Autodesk Inventor part; units mm, degrees
ref_plane "YZ Plane" through (0, 0, 0) normal (1, 0, 0) x (0, 1, 0)
ref_plane "XZ Plane" through (0, 0, 0) normal (0, 1, 0) x (-1, 0, 0)
ref_plane "XY Plane" through (0, 0, 0) normal (0, 0, 1) x (1, 0, 0)
sketch "Sketch1" plane through (0, 0, 0) normal (0, 1, 0) x (-1, 0, 0)
  line L0 (-25, -25) -> (25, -25)
  line L1 (25, -25) -> (25, 25)
  line L2 (25, 25) -> (-25, 25)
  line L3 (-25, 25) -> (-25, -25)
  line L4 (-25, -25) -> (25, 25) construction
  line L5 (25, -25) -> (-25, 25) construction
  point P0 (0, 0)
  dimension "d0" = 50
  dimension "d1" = 50
extrude "Extrusion1" add sketch "Sketch1" along normal blind 1
sketch "Sketch2" plane through (0, 1, 0) normal (0, 1, 0) x (1, 0, 0)
  line L0 (25, -25) -> (25, -15)
  line L1 (25, -25) -> (25, 25)
  line L2 (25, -15) -> (23.4, -15)
  line L3 (23.4, -15) -> (23.4, -5)
  line L4 (23.4, -5) -> (25, -5)
  line L5 (25, -5) -> (25, 5)
  line L6 (25, 5) -> (23.4, 5)
  line L7 (23.4, 5) -> (23.4, 15)
  line L8 (23.4, 15) -> (25, 15)
  line L9 (25, 15) -> (25, 25)
  line L10 (27, 25) -> (27, -25)
  line L11 (27, -25) -> (25, -25)
  point P0 (0, 0)
  dimension "d4" = 1.6
  dimension "d5" = 10
  dimension "d6" = 10
extrude "Extrusion2" cut sketch "Sketch2" against normal blind 1
sketch "Sketch3" plane through (0, 1, 0) normal (0, 1, 0) x (1, 0, 0)
  line L0 (25, 25) -> (25, 24)
  line L1 (25, 24) -> (15, 24)
  line L2 (15, 24) -> (15, 25)
  line L3 (25, 25) -> (-25, 25)
  line L4 (15, 25) -> (5, 25)
  line L5 (5, 25) -> (5, 24)
  line L6 (5, 24) -> (-5, 24)
  line L7 (-5, 24) -> (-5, 25)
  line L8 (-5, 25) -> (-15, 25)
  line L9 (-15, 25) -> (-15, 24)
  line L10 (-15, 24) -> (-25, 24)
  line L11 (-25, 24) -> (-25, 27)
  line L12 (-25, 27) -> (25, 27)
  line L13 (25, 27) -> (25, 25)
  point P0 (0, 0)
extrude "Extrusion3" cut sketch "Sketch3" against normal blind 1
sketch "Sketch4" plane through (0, 1, 0) normal (0, 1, 0) x (1, 0, 0)
  line L0 (-25, -25) -> (-25, -15)
  line L1 (-25, -15) -> (-24, -15)
  line L2 (-24, -15) -> (-24, -5)
  line L3 (-24, -5) -> (-25, -5)
  line L4 (-25, 24) -> (-25, -25)
  line L5 (-25, -5) -> (-25, 5)
  line L6 (-25, 24) -> (-25, -25)
  line L7 (-25, 5) -> (-24, 5)
  line L8 (-24, 5) -> (-24, 15)
  line L9 (-24, 15) -> (-25, 15)
  line L10 (-25, 24) -> (-27, 23)
  line L11 (-27, 23) -> (-27, -24.2648)
  line L12 (-27, -24.2648) -> (-25, -25)
  point P0 (0, 0)
  dimension "d11" = 10
  dimension "d12" = 10
  dimension "d13" = 10
extrude "Extrusion4" cut sketch "Sketch4" against normal blind 1 contours L4 L3 L2 L1 | L4 L9 L8 L7
sketch "Sketch5" plane through (0, 1, 0) normal (0, 1, 0) x (1, 0, 0)
  line L0 (-25, -25) -> (-15, -25)
  line L1 (-25, -25) -> (25, -25)
  line L2 (-15, -25) -> (-15, -24)
  line L3 (-15, -24) -> (-5, -24)
  line L4 (-5, -24) -> (-5, -25)
  line L5 (-5, -25) -> (5, -25)
  line L6 (5, -25) -> (5, -24)
  line L7 (5, -24) -> (15, -24)
  line L8 (15, -24) -> (15, -25)
  line L9 (25, -25) -> (25, -26)
  line L10 (25, -26) -> (-25, -26)
  line L11 (-25, -26) -> (-25, -25)
  point P0 (0, 0)
  dimension "d16" = 10
extrude "Extrusion5" cut sketch "Sketch5" against normal blind 1 contours L2 L3 L4 L1 | L6 L7 L8 L1
sketch "Sketch6" plane through (0, 1, 0) normal (0, 1, 0) x (1, 0, 0)
  circle A0 centre (-21.5, -18.2) radius 0.5
  circle A1 centre (-18.2, 21.5) radius 0.5
  circle A2 centre (18.2, -21.5) radius 0.5
  circle A3 centre (21.5, 18.2) radius 0.5
  line L0 (15, -25) -> (25, -25)
  line L1 (25, -25) -> (25, -15)
  line L2 (-25, -25) -> (-15, -25)
  line L3 (-25, -15) -> (-25, -25)
  line L4 (-5, 25) -> (-15, 25)
  line L5 (-25, 24) -> (-25, 15)
  line L6 (25, 24) -> (15, 24)
  line L7 (25, 15) -> (25, 24)
  point P0 (0, 0)
  dimension "d21" = 1
  dimension "d22" = 1
  dimension "d23" = 1
  dimension "d24" = 1
  dimension "d25" = 3.5
  dimension "d26" = 6.8
  dimension "d27" = 6.8
  dimension "d28" = 3.5
  dimension "d29" = 3.5
  dimension "d30" = 6.8
  dimension "d31" = 5.8
  dimension "d32" = 3.5
extrude "Extrusion6" cut sketch "Sketch6" against normal blind 1
sketch "Sketch7" plane through (0, 1, 0) normal (0, 1, 0) x (1, 0, 0)
  line L0 (15.2, 3.55) -> (23.4, 3.55)
  line L1 (23.4, 3.55) -> (23.4, 6.25)
  line L2 (23.4, 6.25) -> (15.2, 6.25)
  line L3 (15.2, 6.25) -> (15.2, 3.55)
  line L4 (23.4, -15) -> (23.4, -5)
  line L5 (15, -25) -> (25, -25)
  line L6 (23.4, 3.55) -> (25, 3.55)
  line L7 (25, 3.55) -> (25, 5)
  line L8 (25, 5) -> (23.4, 5)
  line L9 (23.4, 5) -> (23.4, 3.55)
  point P0 (0, 0)
  dimension "d37" = 8.2
  dimension "d38" = 2.7
  dimension "d39" = 0
  dimension "d40" = 28.55
extrude "Extrusion8" cut sketch "Sketch7" against normal blind 10
properties part number "Side Panel" material "ABS Plastic"
Design review of the part built by this model. Coordinates are the model's own, in mm. Coordinates: 2 decimals unless noted, no trailing zeros. Loops run counter-clockwise (first coordinate to the right, second up) from the corner with the lowest first, then second, coordinate; pieces in that order, holes last. Notation, with made-up numbers: (39.25, -1) - (69.25, -1) arc R20 cw to (69.25, 22) - close; hole circle Ø8 at (-23.5, 62). An arc over 180 degrees is marked (long way). Use CSV: the item, a comma, the result in double quotes. Start each with the question number.
1) Consider section A-A on y = 0.2. Give the number of separate pieces and of enclosed holes in the cut face, then the cut area to 3 significant figures.
2) Wall thickness on L1, parallel to Z at x = 18.2, y = 0.5; L2, parallel to Z at x = 21.5, y = 0.35; L3, parallel to X at y = 0.7, z = 18.2: over which ranges is each line inside the solid? List them lowest first. Write a range as from..to.
3) Consider section C-C on x = 7. Write out the cut boundary in (y, z).
4) For pin 1 Ø0.5 at (y, z) = (0.5, -4.5) entering from +X, flat-tipped, find the tip position at first contact; note if it passes through.
5) Consider section B-B on z = 12.5. Write out the cut boundary in (x, y).
Geometry says:
1,separate pieces,"1"
1,enclosed holes,"4"
1,area,"2,370 mm^2"
2,L1,"-24..-6.25, -3.55..21, 22..25"
2,L2,"-24..-18.7, -17.7..-6.25, -3.55..25"
2,L3,"-25..-22, -21..25"
3,outline,"(0, -25) - (1, -25) - (1, 24) - (0, 24) - close"
4,pin 1,"x = 15.2"
5,outline,"(-24, 0) - (23.4, 0) - (23.4, 1) - (-24, 1) - close"
